Part model, mm, in its own coordinate system. Round coordinates to 2 decimals unless told otherwise and drop trailing zeros. Order: outer loops, then holes, each group sorted by start corner. A loop starts at its lowest first (then second) coordinate and runs counter-clockwise, first axis right, second up. Notation, with made-up numbers: (76.25, -37) - (82.25, -37) arc R20 cw to (82.25, -15) - close; hole circle Ø1 at (27.5, -37). An arc over 180 degrees is marked (long way). Return JSON: item names as keys, results as strings. Group by question number.
Item 1: Saw through at A-A on z = 1.1. List the corners of the cut face in (x, y).
Item 2: Saw through at B-B on y = -1. List the corners of the cut face in (x, z).
Item 3: Saw through at C-C on x = 1. List the corners of the cut face in (y, z).
Item 4: Drop flat-ended pins along their axis: pin 1 (0.9 mm diameter, centred on y = -27, z = 1.5, fed in from +X); pin 2 (0.9 mm diameter, centred on x = 2.5, z = 1.5, fed in from -Y); pin 3 (1.5 mm diameter, centred on y = -27, z = 1.5, fed in from -X). Give the stop position or say it passes through.
Item 5: Probe probe 1 along X at (y, z) = (-3, 2.7); probe 2 along Y at (x, z) = (59.5, 2); probe 3 along Y at (x, z) = (-24.5, 2.35). List the from-to ranges inside material, lowest first.
Autodesk Inventor part; units mm, degrees
ref_plane "YZ Plane" through (0, 0, 0) normal (1, 0, 0) x (0, 1, 0)
ref_plane "XZ Plane" through (0, 0, 0) normal (0, 1, 0) x (-1, 0, 0)
ref_plane "XY Plane" through (0, 0, 0) normal (0, 0, 1) x (1, 0, 0)
sketch "Sketch1" plane through (0, 0, 0) normal (0, 0, 1) x (1, 0, 0)
  circle A0 centre (0, 0) radius 85 construction
  line L0 (-64.8074, 55) -> (64.8074, 55) construction
  line L1 (64.8074, -25) -> (-64.8074, -25)
  line L2 (-64.8074, -25) -> (-64.8074, 25)
  line L3 (-64.8074, 25) -> (64.8074, 25)
  line L4 (64.8074, 25) -> (64.8074, -25)
  line L5 (64.8074, -25) -> (-64.8074, 25) construction
  line L6 (-64.8074, -25) -> (64.8074, 25) construction
  dimension "d0" = 170
  dimension "d1" = 55
  dimension "d2" = 129.6148
  dimension "d3" = 50
extrude "Extrusion1" add sketch "Sketch1" along normal blind 3
sketch "Sketch2" plane through (0, 0, 3) normal (0, 0, 1) x (1, 0, 0)
  line L0 (-64.8074, -25) -> (64.8074, -25)
  line L1 (-40, -25) -> (-60, -25)
  line L2 (-60, -25) -> (-60, -28)
  line L3 (-60, -28) -> (-40, -28)
  line L4 (-40, -28) -> (-40, -25)
  line L5 (-20, -25) -> (-10, -25)
  line L6 (-10, -25) -> (-10, -28)
  line L7 (-10, -28) -> (-20, -28)
  line L8 (-20, -28) -> (-20, -25)
  point P0 (0, 0)
  dimension "d6" = 20
  dimension "d7" = 3
  dimension "d8" = 10
  dimension "d9" = 3
  dimension "d10" = 10
  dimension "d11" = 20
extrude "Extrusion2" add sketch "Sketch2" against normal blind 3
sketch "Sketch3" plane through (0, 0, 3) normal (0, 0, 1) x (1, 0, 0)
  line L0 (-60, 10) -> (-57, 10)
  line L1 (-57, 10) -> (-57, -10)
  line L2 (-57, -10) -> (-60, -10)
  line L3 (-60, -10) -> (-60, 10)
  point P0 (0, 0)
  point P1 (-60, 0)
  dimension "d14" = 3
  dimension "d15" = 20
  dimension "d16" = 57
extrude "Extrusion3" cut sketch "Sketch3" against normal blind 3
mirror "Mirror1" about plane through (0, 0, 0) normal (1, 0, 0) of "Extrusion2", "Extrusion3"
properties part number "Frount plate"
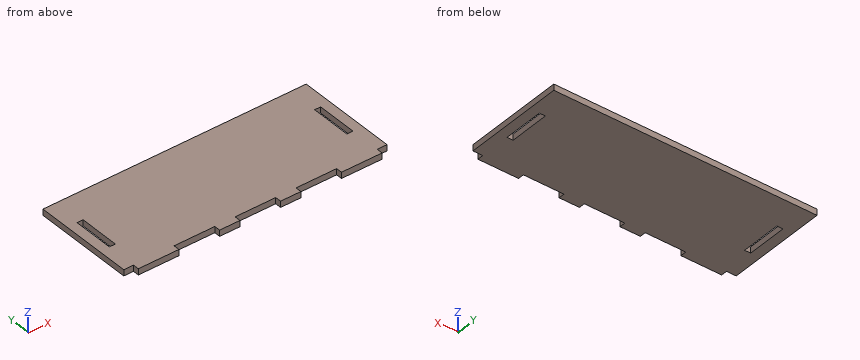
Filled in:
{
 "1": {"outline": "(-64.81, -25) - (-60, -25) - (-60, -28) - (-40, -28) - (-40, -25) - (-20, -25) - (-20, -28) - (-10, -28) - (-10, -25) - (10, -25) - (10, -28) - (20, -28) - (20, -25) - (40, -25) - (40, -28) - (60, -28) - (60, -25) - (64.81, -25) - (64.81, 25) - (-64.81, 25) - close; hole (-60, -10) - (-57, -10) - (-57, 10) - (-60, 10) - close; hole (57, -10) - (60, -10) - (60, 10) - (57, 10) - close"},
 "2": {"outline": "(-64.81, 0) - (-60, 0) - (-60, 3) - (-64.81, 3) - close; (-57, 0) - (57, 0) - (57, 3) - (-57, 3) - close; (60, 0) - (64.81, 0) - (64.81, 3) - (60, 3) - close"},
 "3": {"outline": "(-25, 0) - (25, 0) - (25, 3) - (-25, 3) - close"},
 "4": {"pin 1": "stops at x = 60", "pin 2": "stops at y = -25", "pin 3": "stops at x = -60"},
 "5": {"probe 1": "x = -64.81 to -60, -57 to 57, 60 to 64.81", "probe 2": "y = -28 to -10, 10 to 25", "probe 3": "y = -25 to 25"}
}
